Job drawing, mm, ordinate dimensions from the low corner. One solid piece. A direction names the side the tool comes from. Coordinates: 2 decimals unless noted, no trailing zeros. Loops run counter-clockwise (first coordinate to the right, second up) from the corner with the lowest first, then second, coordinate; pieces in that order, holes last. Notation, with made-up numbers: (86.5, 51.25) -> (132.5, 51.25) arc R21 ccw to (132.5, 65.25) -> close; hole circle Ø11 at (-9.75, -24.5). An arc over 180 degrees is marked (long way). Use one line per item in the form item = value. Start each with the question number.
(1) 3-axis set-ups, long thin cutter, end or side, ignore diameter. For the marked faces 1, 2 and 3: which of +Z, -Z, +X, -X, +Y, -Y reach the whole face in a straight line?
(2) Band-saw the part on D-D on y = 27.5. Give the cut face in (x, z), then the cut area to 3 significant figures.
(3) Pin check, flat tips, straight feed: P1, Ø2.5, axis at x = 57, z = 7.5, coming from the -Y side; P2, Ø7.5, axis at x = 10, z = 6.5, coming from the +Y side; P3, Ø6, axis at y = 10, z = 10, coming from the -X side; P4, Ø6, axis at y = 29.5, z = 13, coming from the +X side. Stop position of each tip, or through.
(4) Band-saw the part on C-C on z = 13.5. Give the cut face in (x, y), then the cut area to 3 significant figures.
(5) Drill centre lines: L1, parallel to X at y = 2.95, z = 7.5; L2, parallel to X at y = 3, z = 12.25; L3, parallel to Z at x = 7, y = 1. Where is each one in solid material? Low to high. Write a range as [from, to].
(6) Band-saw the part on A-A on z = 7.5. Give the cut face in (x, y), then the cut area to 3 significant figures.
(7) Mould opens along X. For the marked faces 4, 5 and 6 say: +X half, -X half, draft (parallel to the pull), parting line (faces both ways), or undercut.
(8) Band-saw the part on B-B on x = 7. Give the cut face in (y, z), then the cut area to 3 significant figures.
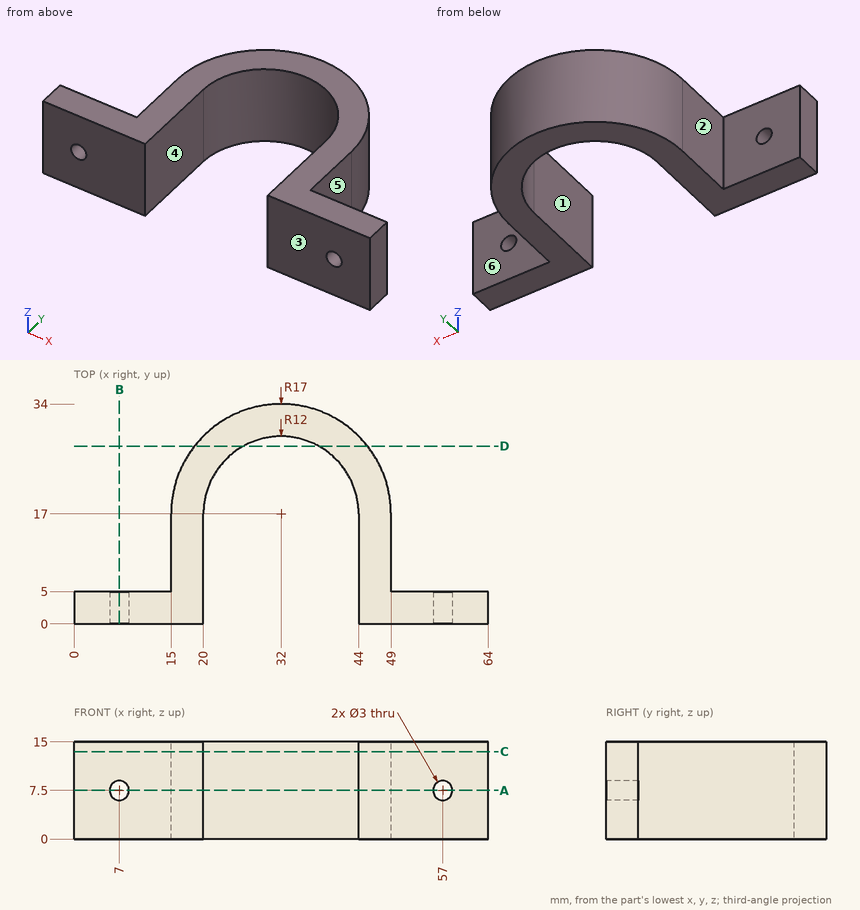
A:
q1.face_1 = +Z, -Z, -Y
q1.face_2 = +Z, -Z, -X, +Y
q1.face_3 = +Z, -Z, +X, -X, -Y
q2.outline = (18.63, 0) -> (26.19, 0) -> (26.19, 15) -> (18.63, 15) -> close; (37.81, 0) -> (45.37, 0) -> (45.37, 15) -> (37.81, 15) -> close
q2.area = 227 mm²
q3.P1 = through
q3.P2 = 5
q3.P3 = 15
q3.P4 = 46.1
q4.outline = (0, 0) -> (20, 0) -> (20, 17) arc R12 cw to (44, 17) -> (44, 0) -> (64, 0) -> (64, 5) -> (49, 5) -> (49, 17) arc R17 ccw to (15, 17) -> (15, 5) -> (0, 5) -> close
q4.area = 548 mm²
q5.L1 = [0, 5.5], [8.5, 20], [44, 55.5], [58.5, 64]
q5.L2 = [0, 20], [44, 64]
q5.L3 = [0, 6], [9, 15]
q6.outline = (0, 0) -> (5.5, 0) -> (5.5, 5) -> (0, 5) -> close; (8.5, 0) -> (20, 0) -> (20, 17) arc R12 cw to (44, 17) -> (44, 0) -> (55.5, 0) -> (55.5, 5) -> (49, 5) -> (49, 17) arc R17 ccw to (15, 17) -> (15, 5) -> (8.5, 5) -> close; (58.5, 0) -> (64, 0) -> (64, 5) -> (58.5, 5) -> close
q6.area = 518 mm²
q7.face_4 = undercut
q7.face_5 = +X half
q7.face_6 = draft
q8.outline = (0, 0) -> (5, 0) -> (5, 6) -> (0, 6) -> close; (0, 9) -> (5, 9) -> (5, 15) -> (0, 15) -> close
q8.area = 60.0 mm²
